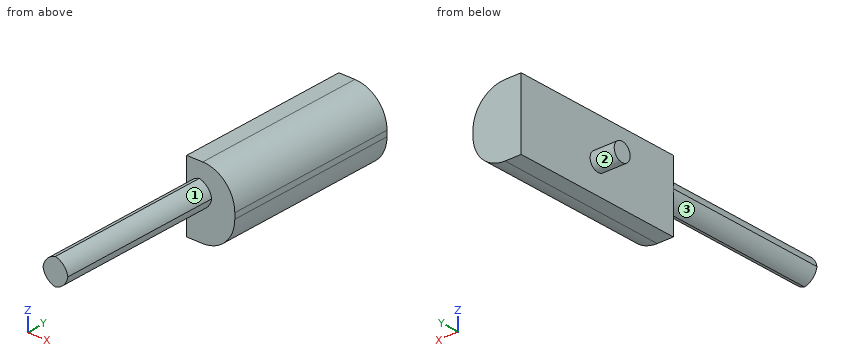
from build123d import *

# Parameters (mm, degrees)
F0_W        = 39.7763997316
F0_H        = 4.2672008276
F1_DEPTH    = 4
F2_T1_DEPTH = 52.4763997316
F3_W        = 27.6340441778
F3_H        = 11.0536180437
F4_DEPTH    = 7.62
F5_R        = 5.08
F6_R        = 1.45
F7_DEPTH    = 3.81


# Not quite as in the source:
# - a fillet or chamfer that OpenCascade refuses, or shapes differently, is made with other operations: its cross-section is extruded or revolved along the edge and cut away or added


with BuildPart() as f1:
    # F0 (on Right) → F1 (new body)
    with BuildSketch(Plane.YZ):
        with Locations((-19.8881998658, 24.0791998804)):
            Rectangle(F0_W, F0_H)
    extrude(amount=F1_DEPTH)

    # F2: fillet of radius 2.54 on 4 edges, made by hand

    # F2_s2 → F2_t1 (cut)
    with BuildSketch(Plane.XZ.offset(-6.35)):
        with BuildLine():
            ThreePointArc((1.46, 26.2128002942), (3.2560512242, 25.4688515184), (4, 23.6728002942))
            Line((4, 23.6728002942), (4, 26.2128002942))
            Line((4, 26.2128002942), (1.46, 26.2128002942))
        make_face()
        with BuildLine():
            ThreePointArc((2.54, 26.2128002942), (0.7439487758, 25.4688515184), (0, 23.6728002942))
            Line((0, 23.6728002942), (0, 26.2128002942))
            Line((0, 26.2128002942), (2.54, 26.2128002942))
        make_face()
        with BuildLine():
            ThreePointArc((1.46, 21.9455994666), (3.2560512242, 22.6895482423), (4, 24.4855994666))
            Line((4, 24.4855994666), (4, 21.9455994666))
            Line((4, 21.9455994666), (1.46, 21.9455994666))
        make_face()
        with BuildLine():
            ThreePointArc((2.54, 21.9455994666), (0.7439487758, 22.6895482423), (0, 24.4855994666))
            Line((0, 24.4855994666), (0, 21.9455994666))
            Line((0, 21.9455994666), (2.54, 21.9455994666))
        make_face()
    extrude(amount=F2_T1_DEPTH, mode=Mode.SUBTRACT)

    # F3 (on Right) → F4 (join)
    with BuildSketch(Plane.YZ):
        with Locations((0.1553441398, 23.0435747653)):
            Rectangle(F3_W, F3_H)
    extrude(amount=F4_DEPTH)

    # F5
    f5_edges = [f1.edges().sort_by_distance(p)[0] for p in [
        (7.62, 0.155344, 28.570384),
        (7.62, 0.155344, 17.516766),
    ]]
    fillet(f5_edges, radius=F5_R)

    # F6 (on face) → F7 (join)
    with BuildSketch(Plane(origin=(0, 0, 0), x_dir=(0, -1, 0), z_dir=(-1, 0, 0))):
        with Locations((0, 22.1642478059)):
            Circle(F6_R)
    extrude(amount=F7_DEPTH)


solid = f1.part
Geometry: final body of the model. Coordinates: model frame, mm. Face numbers are marked on the shaded views. A direction names the side the tool comes from. Give positions to 0.01 mm unless a question says otherwise; leave off trailing zeros. Loops run counter-clockwise (first coordinate to the right, second up) from the corner with the lowest first, then second, coordinate; pieces in that order, holes last. Notation, with made-up numbers: (33.5, 7) - (55.5, 7) arc R6 cw to (55.5, 14) - close; hole circle Ø1 at (27.5, 37.5). An arc over 180 degrees is marked (long way). One line per question, with ' | ' between items. Start each with the question number.
(1) Ray query, line 1 (Y direction, x = 0.25, z = 19.5); line 2 (Z direction, x = 2.75, y = -5); line 3 (X direction, y = 10.5, z = 27.25). Return the intervals inside material, ascending. Write a range as from..to.
(2) Section query C-C on z = 21.25. Return loops of the section in (x, y).
(3) Section query B-B on x = 0.5. Return loops of the section in (y, z), then the cut area to 3 significant figures.
(4) Section query A-A on y = 0. Return loops of the section in (x, z), then the cut area to 3 significant figures.
(5) Contact query for flat-ended pins moving along their axis: pin 1 (1 mm diameter, centred on y = -29, z = 26, fed in from +X); pin 2 (2 mm diameter, centred on x = 4, y = -26, fed in from -Z); pin 3 (5 mm diameter, centred on y = 1, z = 27.5, fed in from +X); pin 4 (1 mm diameter, centred on x = 1.5, y = -14, fed in from +Z). Output: stop coordinate, or through.
(6) Reachability of the marked faces 1, 2 and 3 from +Z, -Z, +X, -X, +Y, -Y: full face, straight path, thin tool, end or side. Return the list, or none.
(7) Section query D-D on x = 5.25. Return loops of the section in (y, z), then the cut area to 3 significant figures.
The answers:
1) line 1: -13.66..13.97 | line 2: 17.52..28.57 | line 3: 0..5.96
2) outline: (-3.81, -1.13) - (0, -1.13) - (0, -13.66) - (7.44, -13.66) - (7.44, 13.97) - (0, 13.97) - (0, 1.13) - (-3.81, 1.13) - close
3) outline: (-39.78, 22.97) - (-13.66, 22.97) - (-13.66, 17.52) - (13.97, 17.52) - (13.97, 28.57) - (-13.66, 28.57) - (-13.66, 25.19) - (-39.78, 25.19) - close | area: 363 mm2
4) outline: (-3.81, 20.71) - (0, 20.71) - (0, 17.52) - (2.54, 17.52) arc R5.08 ccw to (7.62, 22.6) - (7.62, 23.49) arc R5.08 ccw to (2.54, 28.57) - (0, 28.57) - (0, 23.61) - (-3.81, 23.61) - close | area: 84.2 mm2
5) pin 1: x = 3.22 | pin 2: z = 22.47 | pin 3: x = 7.39 | pin 4: z = 28.57
6) face 1: +Z, +X, -Y | face 2: -X | face 3: -Z, -X, -Y
7) outline: (-13.66, 18.3) - (13.97, 18.3) - (13.97, 27.79) - (-13.66, 27.79) - close | area: 262 mm2
